Drawing for the job (mm, zero at the part's lowest x, y, z). Round coordinates to 2 decimals unless told otherwise and drop trailing zeros. Loops run counter-clockwise (first coordinate to the right, second up) from the corner with the lowest first, then second, coordinate; pieces in that order, holes last. Notation, with made-up numbers: M 84.25,62.25 L 90.25,62.25 A11 ccw 90.25,66.25 Z; hole C -0.75,-5.75 d10. An arc over 180 degrees is marked long. Write each question's results on one line, items separated by ' | '.
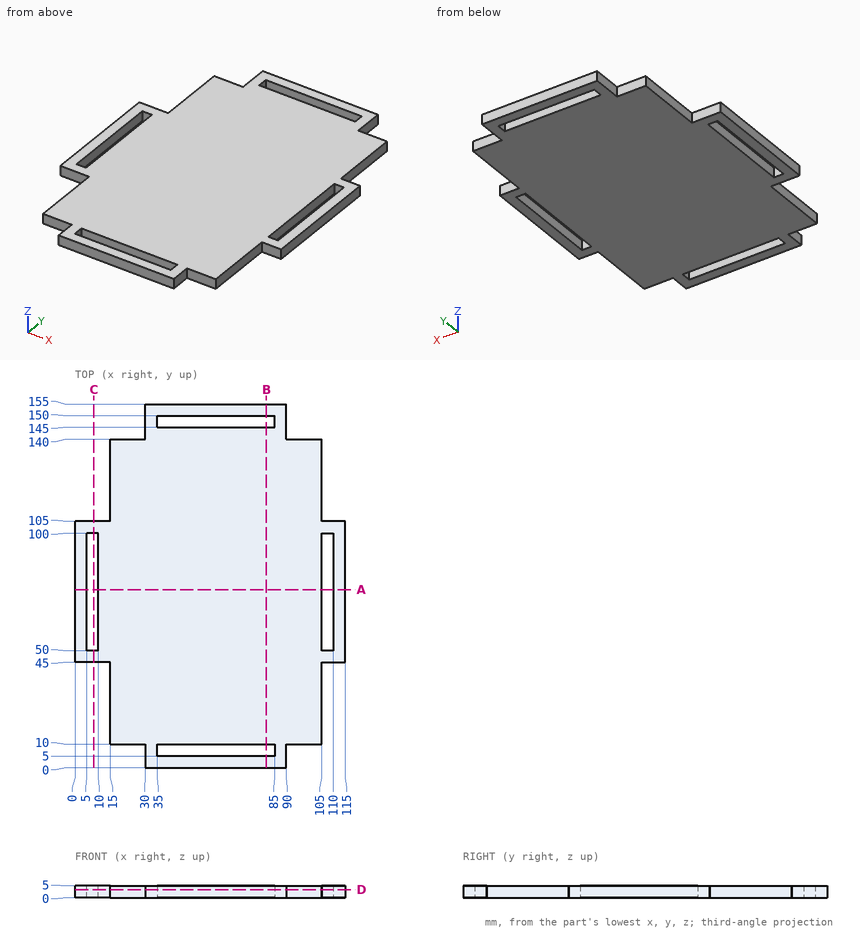
Item 1: Band-saw the part on C-C on x = 8. Give the cut face in (y, z).
Filled sheet:
outline: M 45,0 L 50,0 L 50,5 L 45,5 Z; M 100,0 L 105,0 L 105,5 L 100,5 Z
Item 2: Band-saw the part on A-A on y = 76. Give the cut face in (x, z).
Filled sheet:
outline: M 0,0 L 5,0 L 5,5 L 0,5 Z; M 10,0 L 105,0 L 105,5 L 10,5 Z; M 110,0 L 115,0 L 115,5 L 110,5 Z
Item 3: Drop flat-ended pins along their axis: P1, Ø2.5, axis at y = 66, z = 3, coming from the -X side; P2, Ø1, axis at y = 39.5, z = 2, coming from the -X side; P3, Ø1.5, axis at y = 125, z = 2, coming from the +X side; P4, Ø1.5, axis at x = 108, z = 1.5, coming from the +Y side. Give the stop position or say it passes through.
Filled sheet:
P1: x = 0 | P2: x = 15 | P3: x = 105 | P4: y = 105
Item 4: Wall check: L1, parallel to Y at x = 51.5, z = 2.1; L2, parallel to Y at x = 7, z = 2; L3, parallel to X at y = 87, z = 1.05. Give the ranges that are in metal, low to high.
Filled sheet:
L1: 0 to 5, 10 to 145, 150 to 155 | L2: 45 to 50, 100 to 105 | L3: 0 to 5, 10 to 105, 110 to 115
Item 5: Band-saw the part on B-B on x = 81.5. Give the cut face in (y, z), and give its area (3 significant figures).
Filled sheet:
outline: M 0,0 L 5,0 L 5,5 L 0,5 Z; M 10,0 L 145,0 L 145,5 L 10,5 Z; M 150,0 L 155,0 L 155,5 L 150,5 Z | area: 725 mm^2
Item 6: Band-saw the part on D-D on z = 3.45. Count the separate pieces of the cut face and the enclosed holes in it, and give its area (3 significant figures).
Filled sheet:
separate pieces: 1 | enclosed holes: 4 | area: 13,700 mm^2
